Read the model definition and answer for the solid it produces. Units are mm, in the model's axes. A direction names the side the tool comes from. Round coordinates to 2 decimals unless told otherwise and drop trailing zeros. Loops run counter-clockwise (first coordinate to the right, second up) from the corner with the lowest first, then second, coordinate; pieces in that order, holes last. Notation, with made-up numbers: (-36.75, 65.25) -> (-17.75, 65.25) arc R36 cw to (-17.75, 100.25) -> close; hole circle Ø3 at (-29.75, 53.25). An arc over 180 degrees is marked (long way). Put each result on its own line as item: value.
from build123d import *

# Parameters (mm, degrees)
F1_DEPTH = 530
F3_DEPTH = 25
F4_R     = 7
F5_DEPTH = 5.001
F7_DEPTH = 1060.001
F8_DEPTH = 3


# Not quite as in the source:
# - a pattern or mirror of a feature is missing from the dataset's text; its kind, count and spacing are read off the source's solid


with BuildPart() as f1:
    # F0 (on Right) → F1 (new body, symmetric)
    with BuildSketch(Plane.YZ):
        Polygon((0, 940), (0, 0), (-6.4704761276, -24.1481456572), (-1.6408469961, -25.4422408827), (5, -0.6582624879), (5, 941.3397459622), (-13.1698729811, 972.8108891325), (-17.5, 970.3108891325), align=None)
    extrude(amount=F1_DEPTH, both=True)

    # F2 (on face) → F3 (cut)
    with BuildSketch(Plane.YZ.offset(530)):
        Polygon((5, 0), (0, 0), (-6.4704761276, -24.1481456572), (-1.6408469961, -25.4422408827), (5, -0.6582624879), align=None)
        Polygon((-17.5, 970.3108891325), (0, 940), (5, 940), (5, 941.3397459622), (-13.1698729811, 972.8108891325), align=None)
    f3 = extrude(amount=-F3_DEPTH, mode=Mode.SUBTRACT)

    # F3_copies: F3 across plane
    add(f3.mirror(Plane(origin=(0, 0, 0), x_dir=(0, 0, -1), z_dir=(-1, 0, 0))), mode=Mode.SUBTRACT)

    # F4 (on face) → F5 (cut, through all)
    with BuildSketch(Plane.XZ):
        with Locations((0, 30)):
            Circle(F4_R)
        with Locations((110, 30)):
            Circle(F4_R)
        with Locations((220, 30)):
            Circle(F4_R)
        with Locations((330, 30)):
            Circle(F4_R)
        with Locations((440, 30)):
            Circle(F4_R)
        with Locations((-110, 30)):
            Circle(F4_R)
        with Locations((-220, 30)):
            Circle(F4_R)
        with Locations((-330, 30)):
            Circle(F4_R)
        with Locations((-440, 30)):
            Circle(F4_R)
    extrude(amount=-F5_DEPTH, mode=Mode.SUBTRACT)

    # F6 (on face) → F7 (cut, through all)
    with BuildSketch(Plane.YZ.offset(530)):
        Polygon((0, 12), (0, 0), (-6.4704761276, -24.1481456572), (-1.6408469961, -25.4422408827), (5, -0.6582624879), (5, 12), align=None)
    extrude(amount=-F7_DEPTH, mode=Mode.SUBTRACT)

    # F8 (add): faces of the model
    f8_faces = [f1.faces().sort_by_distance(p)[0] for p in [
        (0, 5, 477.2673971314),
        (0, -4.0849364905, 957.0753175473),
    ]]
    extrude(f8_faces, amount=F8_DEPTH, dir=(0, 1, 0))


solid = f1.part
Item 1: The part is cut by section A-A (x = -363). Determine the outline of the cut face in (y, z), then the cut area to 3 significant figures.
Derived:
outline: (-17.5, 970.31) -> (0, 940) -> (0, 12) -> (8, 12) -> (8, 941.34) -> (-10.17, 972.81) -> (-13.17, 972.81) -> close
area: 7,700 mm^2
Item 2: The part is cut by section B-B (z = 700.5). Determine the outline of the cut face in (x, y).
Derived:
outline: (-530, 0) -> (530, 0) -> (530, 8) -> (-530, 8) -> close
Item 3: Which of the six approach directions +Z, -Z, +X, -X, +Y, -Y give full straight-line access (tool end or side, diameter ignored) to faces 4 (the flat face through (7, 0, 482)), 5 (the flat face through (-505, -6, 956)), 6 (the flat face through (7, 8, 470))?
Derived:
face 4: -Z, +X, -X, -Y
face 5: +Z, -X, +Y, -Y
face 6: +Z, -Z, +X, -X, +Y
Item 4: For a pull along Z with two mould halves and no side action, classify faces 1 (the flat face through (7.07, -8.872, 955.368)), 2 (the flat face through (505, -6, 956)), 3 (the flat face through (7.07, -0.96, 956.86)) as pulls with the +Z half, pulls with the -Z half, needs draft (parallel to the pull), parting line crosses it, or undercut.
Derived:
face 1: pulls with the -Z half
face 2: needs draft
face 3: pulls with the +Z half
Item 5: Flat-ended cylindrical pins translate along their axes: pin 1 Ø10 at (x, z) = (421.5, 392.5) entering from -Y; pin 2 Ø7.5 at (y, z) = (-3.5, 962.5) entering from +X; pin 3 Ø9 at (x, y) = (-518.5, 6) entering from +Z. Find the tip coordinate at first contact, or state that the pin passes through.
Derived:
pin 1: stops at y = 0
pin 2: stops at x = 505
pin 3: stops at z = 940
Item 6: Find the intervals of material crossed by line 1 along Y through (x, z) = (93.5, 189.5); line 2 along Z through (x, y) = (-220, 3.5); line 3 along Z through (x, y) = (0, 2.75), in increasing order.
Derived:
line 1: y = 0 to 8
line 2: z = 12 to 23, 37 to 949.13
line 3: z = 12 to 23, 37 to 950.43
Item 7: The part is cut by section C-C (y = -4). Determine the outline of the cut face in (x, z), then the cut area to 3 significant figures.
Derived:
outline: (-505, 946.93) -> (505, 946.93) -> (505, 962.12) -> (-505, 962.12) -> close
area: 15,300 mm^2
